Can you work these out from the model? Positions are in its coordinate system, mm. A direction names the side the tool comes from. Round coordinates to 2 decimals unless told otherwise and drop trailing zeros. Order: outer loops, then holes, each group sorted by start corner. A loop starts at its lowest first (then second) coordinate and runs counter-clockwise, first axis right, second up.
Q1. If we section it at C-C (x = 21.15): Please give me the cut outline in (y, z), plus the area to 3 significant figures.
Q2. For faces 5 (the face through (296, 30, 0)), 6 (the face through (49, 30, -250)), 7 (the face through (501, 30, -199)), which set-ups out of +Z, -Z, +X, -X, +Y, -Y let a thin tool reach every point of the face, with its end or its side?
Q3. If I drill on line 1 (X direction, y = 30, z = -87); line 2 (Z direction, x = 550.5, y = 7); line 3 (Y direction, x = 578.85, z = -114), over which ranges is the centre line in solid material (lowest first)?
Q4. We'd pull the mould along Y, two halves only. Please class faces 1 (the face through (10.094, 40.138, -76.05)), 2 (the face through (563.865, 30.66, -326.05)), 3 (the face through (550, 30, -150)), 4 (the face through (296, 0, -203)): pulls with the +Y half, pulls with the -Y half, needs draft (parallel to the pull), parting line crosses it, or undercut.
Q5. If we section it at D-D (z = -159): Please give me the cut outline in (x, y), plus the area to 3 significant figures.
Q6. If we section it at B-B (z = -116.5): Please give me the cut outline in (x, y), plus the area to 3 significant figures.
Q7. Will this pin go through, and if not, where does the flat tip stop? P1, Ø1.5, axis at y = 10, z = -166.5, coming from the -X side.
Q8. If we section it at A-A (y = 30): Count the separate pieces of the cut face and the enclosed holes in it, plus the area to 3 significant figures.
from build123d import *

# Parameters (mm, degrees)
ESTRUSIONE_ESTRUSIONE1_DEPTH  = 60
TAGLIO_ESTRUSIONE2_DEPTH      = 724.602100605
TAGLIO_ESTRUSIONE2_DEPTH_BACK = 724.602100605
SCHIZZO3_OUTSIDE_W            = 746.72
SCHIZZO3_OUTSIDE_H            = 206.72
SCHIZZO3_OUTSIDE_R            = 15
SCHIZZO4_W                    = 100
SCHIZZO4_H                    = 100
TAGLIO_ESTRUSIONE3_DEPTH      = 724.602100605


with BuildPart() as part:
    # Schizzo1 → Estrusione-Estrusione1 (new body)
    with BuildSketch(Plane(origin=(0, 0, 0), x_dir=(1, 0, 0), z_dir=(0, 1, 0))):
        with BuildLine():
            Line((3, 0), (597, 0))
            ThreePointArc((597, 0), (599.121320344, 0.878679656), (600, 3))
            Line((600, 3), (600, 397))
            ThreePointArc((600, 397), (599.121320344, 399.121320344), (597, 400))
            Line((597, 400), (3, 400))
            ThreePointArc((3, 400), (0.878679656, 399.121320344), (0, 397))
            Line((0, 397), (0, 3))
            ThreePointArc((0, 3), (0.878679656, 0.878679656), (3, 0))
        make_face()
    extrude(amount=ESTRUSIONE_ESTRUSIONE1_DEPTH)

    # Schizzo3 outside → Taglio-Estrusione2 (cut, two sides: drawn at the far end of the back side and taken through both)
    # profile 1 of 3: a face of its own
    with BuildSketch(Plane.XY.offset(-TAGLIO_ESTRUSIONE2_DEPTH_BACK)):
        with Locations((300, 30)):
            Rectangle(SCHIZZO3_OUTSIDE_W, SCHIZZO3_OUTSIDE_H)
        with BuildLine():
            Line((3, 60), (597, 60))
            ThreePointArc((597, 60), (599.121320344, 59.121320344), (600, 57))
            Line((600, 57), (600, 3))
            ThreePointArc((600, 3), (599.121320344, 0.878679656), (597, 0))
            Line((597, 0), (3, 0))
            ThreePointArc((3, 0), (0.878679656, 0.878679656), (0, 3))
            Line((0, 3), (0, 57))
            ThreePointArc((0, 57), (0.878679656, 59.121320344), (3, 60))
        make_face(mode=Mode.SUBTRACT)
    # profile 2 of 3: a face of its own
    with BuildSketch(Plane.XY.offset(-TAGLIO_ESTRUSIONE2_DEPTH_BACK)):
        with Locations((21.15, 30)):
            Circle(SCHIZZO3_OUTSIDE_R)
    # profile 3 of 3: a face of its own
    with BuildSketch(Plane.XY.offset(-TAGLIO_ESTRUSIONE2_DEPTH_BACK)):
        with Locations((578.85, 30)):
            Circle(SCHIZZO3_OUTSIDE_R)
    extrude(amount=TAGLIO_ESTRUSIONE2_DEPTH + TAGLIO_ESTRUSIONE2_DEPTH_BACK, mode=Mode.SUBTRACT)

    # Schizzo4 → Taglio-Estrusione3 (cut, through all)
    with BuildSketch(Plane(origin=(0, 0, 0), x_dir=(1, 0, 0), z_dir=(0, 1, 0))):
        with Locations((49, 200)):
            Rectangle(SCHIZZO4_W, SCHIZZO4_H)
        with Locations((551, 200)):
            Rectangle(SCHIZZO4_W, SCHIZZO4_H)
    extrude(amount=TAGLIO_ESTRUSIONE3_DEPTH, mode=Mode.SUBTRACT)


solid = part.part
Solution:
1. outline: (0, -400) - (15, -400) - (15, -250) - (0, -250) - close; (0, -150) - (15, -150) - (15, 0) - (0, 0) - close; (45, -400) - (60, -400) - (60, -250) - (45, -250) - close; (45, -150) - (60, -150) - (60, 0) - (45, 0) - close
1. area: 9,000 mm2
2. face 5: +Z, +X, -X, +Y, -Y
2. face 6: -X, +Y, -Y
2. face 7: +X, +Y, -Y
3. line 1: x = 0 to 6.15, 36.15 to 563.85, 593.85 to 600
3. line 2: z = -400 to -250, -150 to 0
3. line 3: y = 0 to 15, 45 to 60
4. face 1: undercut
4. face 2: undercut
4. face 3: needs draft
4. face 4: pulls with the -Y half
5. outline: (99, 0) - (501, 0) - (501, 60) - (99, 60) - close
5. area: 24,100 mm2
6. outline: (0, 3) arc R3 ccw to (3, 0) - (597, 0) arc R3 ccw to (600, 3) - (600, 57) arc R3 ccw to (597, 60) - (3, 60) arc R3 ccw to (0, 57) - close; hole circle Ø30 at (21.15, 30); hole circle Ø30 at (578.85, 30)
6. area: 34,600 mm2
7. P1: stops at x = 99
8. separate pieces: 5
8. enclosed holes: 0
8. area: 202,000 mm2
